```python
from build123d import *

# Parameters (mm, degrees)
SKETCH2_W               = 200.4
SKETCH2_H               = 250
SKETCH2_W_2             = 160.4
SKETCH2_H_2             = 210
BOSS_EXTRUDE1_DEPTH     = 480
SKETCH3_W               = 160.4
SKETCH3_H               = 25
CUT_EXTRUDE1_DEPTH      = 3
CUT_EXTRUDE2_DEPTH      = 535.282171956
CUT_EXTRUDE2_DEPTH_BACK = 535.282171956
SKETCH4_W               = 100
SKETCH4_H               = 25
SKETCH7_R               = 1.5
CUT_EXTRUDE4_DEPTH      = 20


with BuildPart() as part:
    # Sketch2 → Boss-Extrude1 (new, symmetric)
    with BuildSketch(Plane.XY):
        with Locations((37.499423299, 25.044257703)):
            Rectangle(SKETCH2_W, SKETCH2_H)
        with Locations((37.499423299, 25.044257703)):
            Rectangle(SKETCH2_W_2, SKETCH2_H_2, mode=Mode.SUBTRACT)
    extrude(amount=BOSS_EXTRUDE1_DEPTH, both=True)

    # Sketch3 → Cut-Extrude1 (cut)
    with BuildSketch(Plane.XY.offset(480)):
        with Locations((37.499423299, 130.044257703)):
            Rectangle(SKETCH3_W, SKETCH3_H)
    cut_extrude1 = extrude(amount=-CUT_EXTRUDE1_DEPTH, mode=Mode.SUBTRACT)

    # Mirror1: Cut-Extrude1 across plane
    add(cut_extrude1.mirror(Plane.XY), mode=Mode.SUBTRACT)

    # Sketch4 → Cut-Extrude2 (cut, two sides: drawn at the far end of the back side and taken through both)
    with BuildSketch(Plane(origin=(-42.700576701, 0, 0), x_dir=(0, 0, -1), z_dir=(1, 0, 0)).offset(-CUT_EXTRUDE2_DEPTH_BACK)):
        with Locations((410, -47.455742297)):
            Rectangle(SKETCH4_W, SKETCH4_H)
    extrude(amount=CUT_EXTRUDE2_DEPTH + CUT_EXTRUDE2_DEPTH_BACK, mode=Mode.SUBTRACT)

    # Sketch7 → Cut-Extrude4 (cut)
    with BuildSketch(Plane.XZ.offset(99.955742297)):
        with Locations(Location((112.499423299, 0, 0), (0, 0, 270))):
            Circle(SKETCH7_R)
        with Locations(Location((-37.500576701, 0, 0), (0, 0, 270))):
            Circle(SKETCH7_R)
    extrude(amount=-CUT_EXTRUDE4_DEPTH, mode=Mode.SUBTRACT)


solid = part.part
```
The model under review builds one solid part; all positions refer to its coordinate system, in mm. A direction names the side the tool comes from. Round coordinates to 2 decimals unless told otherwise and drop trailing zeros. Loops run counter-clockwise (first coordinate to the right, second up) from the corner with the lowest first, then second, coordinate; pieces in that order, holes last. Notation, with made-up numbers: M -14,-30 L 40,-30 A18 cw 40,3 Z; hole C -25.75,3.5 d1. An arc over 180 degrees is marked long. Put each result on its own line as item: value.
Q1. Machinability: for faces 4 (the flat face through (128, -59.956, -409)), 5 (the flat face through (-42.701, 30, -7)), 6 (the flat face through (-45, 7, -480)), which of the approach directions +Z, -Z, +X, -X, +Y, -Y give a long, thin tool a straight path to every point of the face, cutting with its end or side? Answer none if there is none.
Result set:
face 4: +X, -X
face 5: +Z, -Z
face 6: -Z, +X, -X, +Y, -Y
Q2. For pin 1 (12 mm diameter, centred on x = 110, y = 34, fed in from -Z), flat-tipped, find the tip position at first contact; note if it passes through.
Result set:
pin 1: passes through
Q3. Consider section C-C, the plane z = 269. Give the boundary of the cut face in (x, y), then the cut area to 3 significant figures.
Result set:
outline: M -62.7,-99.96 L 137.7,-99.96 L 137.7,150.04 L -62.7,150.04 Z; hole M -42.7,-79.96 L 117.7,-79.96 L 117.7,130.04 L -42.7,130.04 Z
area: 16,400 mm²
Q4. Mouldability with a two-part tool opening along Z and no side actions: class faces 1 (the flat face through (-45, 7, 480)), 2 (the flat face through (36, -79.956, 7)), 3 (the flat face through (-53, -59.956, -409)) as released by +Z, released by -Z, zero draft, split by the parting line, or undercut.
Result set:
face 1: released by +Z
face 2: zero draft
face 3: undercut
Q5. Consider section A-A, the plane x = 53. Give the boundary of the cut face in (y, z), then the cut area to 3 significant figures.
Result set:
outline: M -99.96,-480 L -79.96,-480 L -79.96,480 L -99.96,480 Z; M 130.04,-477 L 142.54,-477 L 142.54,-480 L 150.04,-480 L 150.04,480 L 142.54,480 L 142.54,477 L 130.04,477 Z
area: 38,300 mm²
Q6. To check wall thickness, follow L1, parallel to X at y = -84.75, z = 0; L2, parallel to Y at x = 49.5, z = 400; L3, parallel to X at y = -1, z = 335.5. State the ranges of each line that lie inside material, in increasing order.
Result set:
L1: x = -62.7 to -39, -36 to 111, 114 to 137.7
L2: y = -99.96 to -79.96, 130.04 to 150.04
L3: x = -62.7 to -42.7, 117.7 to 137.7
Q7. Consider section B-B, the plane y = 58.5. Give the boundary of the cut face in (x, z), then the cut area to 3 significant figures.
Result set:
outline: M -62.7,-480 L -42.7,-480 L -42.7,480 L -62.7,480 Z; M 117.7,-480 L 137.7,-480 L 137.7,480 L 117.7,480 Z
area: 38,400 mm²
